```python
from build123d import *

# Parameters (mm, degrees)
F0_R            = 11
F1_DEPTH        = 2
F3_DEPTH        = 2
F3_COPIES_COUNT = 12
F4_R            = 4
F5_DEPTH        = 4
F7_DEPTH        = 9


# Not quite as in the source:
# - a pattern or mirror of a feature is missing from the dataset's text; its kind, count and spacing are read off the source's solid


with BuildPart() as f1:
    # F0 (on Top) → F1 (new body)
    with BuildSketch(Plane.XY):
        Circle(F0_R)
    extrude(amount=F1_DEPTH)

    # F2 (on face) → F3 (cut)
    with BuildSketch(Plane.XY.offset(2)):
        with BuildLine():
            Line((9.4187261831, 1.2399988261), (5.4529467376, 0.7178940572))
            ThreePointArc((5.4529467376, 0.7178940572), (5.5, 0), (5.4529467376, -0.7178940572))
            Line((5.4529467376, -0.7178940572), (9.4187261831, -1.2399988261))
            ThreePointArc((9.4187261831, -1.2399988261), (9.5, 0), (9.4187261831, 1.2399988261))
        make_face()
    f3 = extrude(amount=-F3_DEPTH, mode=Mode.SUBTRACT)

    # F3_copies: F3 ×12 about axis
    f3_copies_axis = Axis((0, 0, 0), (0, 0, 1))
    for i in range(1, F3_COPIES_COUNT):
        add(f3.rotate(f3_copies_axis, i * 360 / F3_COPIES_COUNT), mode=Mode.SUBTRACT)

    # F4 (on face) → F5 (join)
    with BuildSketch(Plane(origin=(0, 0, 0), x_dir=(1, 0, 0), z_dir=(0, 0, -1))):
        Circle(F4_R)
    extrude(amount=F5_DEPTH)

    # F6 (on face) → F7 (cut)
    with BuildSketch(Plane(origin=(0, 0, -4), x_dir=(1, 0, 0), z_dir=(0, 0, -1))):
        with BuildLine():
            Line((-2.2366269246, -1.6), (2.2366269246, -1.6))
            ThreePointArc((2.2366269246, -1.6), (2.75, 0), (2.2366269246, 1.6))
            Line((2.2366269246, 1.6), (-2.2366269246, 1.6))
            ThreePointArc((-2.2366269246, 1.6), (-2.75, 0), (-2.2366269246, -1.6))
        make_face()
    extrude(amount=-F7_DEPTH, mode=Mode.SUBTRACT)


solid = f1.part
```
Build history of the part. All positions in model axes, mm. Coordinates: 2 decimals unless noted, no trailing zeros. Write each loop counter-clockwise with the first axis right and the second up, starting at its lowest first coordinate (ties: lowest second). Pieces come first, ordered by that corner, then holes.
1. Band-saw the part on B-B, the plane z = -2.7. Give the cut face in (x, y).
Answer block:
outline: circle Ø8 at (0, 0); hole (-2.24, -1.6) - (2.24, -1.6) arc R2.75 ccw to (2.24, 1.6) - (-2.24, 1.6) arc R2.75 ccw to start
2. Pull direction X, two halves, no side cores. Call faces 1 (the cylindrical face through (0, 5.5, 1)), 2 (the flat face through (0, -2, 2)): released by +X, released by -X, zero draft, split by the parting line, or undercut.
Answer block:
face 1: undercut
face 2: zero draft
3. Band-saw the part on D-D, the plane z = 1.2. Give the number of separate pieces and of enclosed holes in the cut face, and give its area (3 significant figures).
Answer block:
separate pieces: 1
enclosed holes: 13
area: 269 mm2
4. Drop flat-ended pins along their axis: pin 1 (1 mm diameter, centred on y = 3, z = -2, fed in from -X); pin 2 (1 mm diameter, centred on y = 4, z = 0, fed in from +X); pin 3 (1 mm diameter, centred on y = -1.5, z = -1, fed in from +X). Give the stop position or say it passes through.
Answer block:
pin 1: stops at x = -3.12
pin 2: stops at x = 10.43
pin 3: stops at x = 3.87
5. Drill centre lines: probe 1 along Y at (x, z) = (-4, 1.45); probe 2 along Y at (x, z) = (-0.5, 1.3); probe 3 along X at (y, z) = (-7.5, 0.65). Where is each one in solid material? Low to high.
Answer block:
probe 1: y = -10.25 to -8.62, -5.21 to 5.21, 8.62 to 10.25
probe 2: y = -10.99 to -9.49, -5.48 to -1.6, 1.6 to 5.48, 9.49 to 10.99
probe 3: x = -8.05 to -5.75, -3.11 to -0.99, 0.99 to 3.11, 5.75 to 8.05
6. Band-saw the part on C-C, the plane y = -6.25. Give the cut face in (x, z).
Answer block:
outline: (-9.05, 0) - (-4.8, 0) - (-4.8, 2) - (-9.05, 2) - close; (-2.59, 0) - (-0.82, 0) - (-0.82, 2) - (-2.59, 2) - close; (0.82, 0) - (2.59, 0) - (2.59, 2) - (0.82, 2) - close; (4.8, 0) - (9.05, 0) - (9.05, 2) - (4.8, 2) - close
7. Band-saw the part on A-A, the plane x = 0. Give the cut face in (y, z), and give its area (3 significant figures).
Answer block:
outline: (-11, 0) - (-9.5, 0) - (-9.5, 2) - (-11, 2) - close; (-5.5, 0) - (-4, 0) - (-4, -4) - (-1.6, -4) - (-1.6, 2) - (-5.5, 2) - close; (1.6, -4) - (4, -4) - (4, 0) - (5.5, 0) - (5.5, 2) - (1.6, 2) - close; (9.5, 0) - (11, 0) - (11, 2) - (9.5, 2) - close
area: 40.8 mm2
